Design review of the part built by this model. Coordinates are the model's own, in mm. A direction names the side the tool comes from. Give positions to 0.01 mm unless a question says otherwise; leave off trailing zeros. Write each loop counter-clockwise with the first axis right and the second up, starting at its lowest first coordinate (ties: lowest second). Pieces come first, ordered by that corner, then holes.
```python
from build123d import *

# Parameters (mm, degrees)
F0_W     = 15.81
F0_H     = 15.81
F0_R     = 2.425
F1_DEPTH = 9.5
F2_DEPTH = 1.85
F4_W     = 13.37
F4_H     = 13.37
F4_R     = 2.535
F5_DEPTH = 8.5
F6_R     = 1.735
F7_DEPTH = 8.5
F8_DEPTH = 8.5


with BuildPart() as f1:
    # F0 (on Top) → F1 (new body)
    with BuildSketch(Plane.XY):
        Rectangle(F0_W, F0_H)
        with Locations((-3.88, -3.88)):
            Circle(F0_R, mode=Mode.SUBTRACT)
        with Locations((3.88, -3.980963)):
            Circle(F0_R, mode=Mode.SUBTRACT)
        with Locations((-3.88, 3.88)):
            Circle(F0_R, mode=Mode.SUBTRACT)
        with Locations((3.88, 3.88)):
            Circle(F0_R, mode=Mode.SUBTRACT)
        with Locations((-3.88, 3.88)):
            Circle(F0_R)
        with Locations((3.88, 3.88)):
            Circle(F0_R)
        with Locations((3.88, -3.980963)):
            Circle(F0_R)
        with Locations((-3.88, -3.88)):
            Circle(F0_R)
    extrude(amount=F1_DEPTH)

    # F0 (on Top) → F2 (join)
    with BuildSketch(Plane.XY):
        with Locations((-3.88, -3.88)):
            Circle(F0_R)
        with Locations((3.88, -3.980963)):
            Circle(F0_R)
        with Locations((3.88, 3.88)):
            Circle(F0_R)
        with Locations((-3.88, 3.88)):
            Circle(F0_R)
    extrude(amount=-F2_DEPTH)

    # F4 (on face) → F5 (cut)
    with BuildSketch(Plane.XY.offset(9.5)):
        Rectangle(F4_W, F4_H)
        Circle(F4_R, mode=Mode.SUBTRACT)
    extrude(amount=-F5_DEPTH, mode=Mode.SUBTRACT)

    # F6 (on face) → F7 (join)
    with BuildSketch(Plane.XY.offset(9.5)):
        Circle(F6_R)
    extrude(amount=-F7_DEPTH)

    # F6 (on face) → F8 (cut)
    with BuildSketch(Plane.XY.offset(9.5)):
        Circle(F6_R)
    extrude(amount=-F8_DEPTH, mode=Mode.SUBTRACT)


solid = f1.part
```
(1) Tool access review of faces 1 (the face through (4, -4, -1.85)), 2 (the face through (5.184, 5.925, -0.912)), 3 (the face through (-3, 0, 1)): name each direction out of +Z, -Z, +X, -X, +Y, -Y from which nothing blocks a thin tool from reaching the whole face with its end or side.
Resolved:
face 1: -Z, +X, -X, +Y, -Y
face 2: -Z
face 3: +Z
(2) To check wall thickness, follow L1, parallel to Y at x = 0, z = 5.25 (3 decimals); L2, parallel to X at y = -4, z = -1.5; L3, parallel to X at y = -6, z = 7.25 (3 decimals). State the ranges of each line that lie inside material, in increasing order.
Resolved:
L1: y = -7.905 to -6.685, -2.535 to -1.735, 1.735 to 2.535, 6.685 to 7.905
L2: x = -6.3 to -1.46, 1.46 to 6.3
L3: x = -7.905 to -6.685, 6.685 to 7.905
(3) Consider section A-A, the plane z = 6.5. Give the boundary of the cut face in (x, y) (3 decimals), then the cut area to 3 significant figures.
Resolved:
outline: (-7.905, -7.905) - (7.905, -7.905) - (7.905, 7.905) - (-7.905, 7.905) - close; circle Ø5.07 at (0, 0); hole (-6.685, -6.685) - (6.685, -6.685) - (6.685, 6.685) - (-6.685, 6.685) - close; hole circle Ø3.47 at (0, 0)
area: 81.9 mm2
(4) Mouldability with a two-part tool opening along Y and no side actions: class faces 4 (the face through (-7.905, 0, 5)), 5 (the face through (0, -6.685, 5)) as pulls with the +Y half, pulls with the -Y half, needs draft (parallel to the pull), parting line crosses it, or undercut.
Resolved:
face 4: needs draft
face 5: undercut
(5) Consider section B-B, the plane y = 3.88. Give the boundary of the cut face in (x, z) (3 decimals), then the cut area to 3 significant figures.
Resolved:
outline: (-7.905, 0) - (-6.305, 0) - (-6.305, -1.85) - (-1.455, -1.85) - (-1.455, 0) - (1.455, 0) - (1.455, -1.85) - (6.305, -1.85) - (6.305, 0) - (7.905, 0) - (7.905, 9.5) - (6.685, 9.5) - (6.685, 1) - (-6.685, 1) - (-6.685, 9.5) - (-7.905, 9.5) - close
area: 54.5 mm2
(6) Consider section C-C, the plane x = 3.88. Give the boundary of the cut face in (y, z) (3 decimals).
Resolved:
outline: (-7.905, 0) - (-6.406, 0) - (-6.406, -1.85) - (-1.556, -1.85) - (-1.556, 0) - (1.455, 0) - (1.455, -1.85) - (6.305, -1.85) - (6.305, 0) - (7.905, 0) - (7.905, 9.5) - (6.685, 9.5) - (6.685, 1) - (-6.685, 1) - (-6.685, 9.5) - (-7.905, 9.5) - close
(7) Clearance check with flat-ended pins moving along their axes: P1, Ø3, axis at x = 0, y = 0, coming from the -Z side; P2, Ø4, axis at x = 4, y = 0.5, coming from the +Z side. State where each tip first meets the part, or that it passes through.
Resolved:
P1: stops at z = 0
P2: stops at z = 9.5
